Verification items for the finished model (mm, model axes). A direction names the side the tool comes from. Give positions to 0.01 mm unless a question says otherwise; leave off trailing zeros. Order: outer loops, then holes, each group sorted by start corner. A loop starts at its lowest first (then second) coordinate and runs counter-clockwise, first axis right, second up. Notation, with made-up numbers: M 3,62 L 24,62 A13 cw 24,72 Z; hole C 29,-13.5 d9. An arc over 180 degrees is marked long. Answer as a JSON object with one key per item and string values.
Autodesk Fusion 360 part; units mm, degrees
sketch "Boceto1" plane through (0, 0, 0) normal (1, 0, 0) x (0, 1, 0)
  line L0 (7.5, 35) -> (-7.5, 35)
  line L1 (-7.5, 35) -> (-7.5, -35)
  line L2 (-7.5, -35) -> (7.5, -35)
  line L3 (7.5, -35) -> (7.5, 35)
  line L4 (7.5, 35) -> (-7.5, -35) construction
  line L5 (-7.5, 35) -> (7.5, -35) construction
  circle A0 centre (0, 30) radius 2
  circle A1 centre (0, -30) radius 2
  line L6 (0, 35) -> (0, -35) construction
  dimension "d1" = 15
  dimension "d2" = 70
  dimension "d3" = 4
  dimension "d4" = 4
  dimension "d5" = 60
  dimension "d6" = 30
extrude "Extruir1" add sketch "Boceto1" along normal blind 3
sketch "Boceto2" plane through (3, 0, 0) normal (1, 0, 0) x (0, 1, 0)
  circle A0 centre (0, 30) radius 2
  circle A1 centre (0, -30) radius 2
  line L0 (7.5, -35) -> (7.5, 35)
  line L1 (7.5, 35) -> (-7.5, 35)
  line L2 (-7.5, 35) -> (-7.5, -35)
  line L3 (-7.5, -35) -> (7.5, -35)
  line L4 (3.25, 20) -> (-3.25, 20)
  line L5 (-3.25, 20) -> (-3.25, -20)
  line L6 (-3.25, -20) -> (3.25, -20)
  line L7 (3.25, -20) -> (3.25, 20)
  line L8 (3.25, 20) -> (-3.25, -20) construction
  line L9 (-3.25, 20) -> (3.25, -20) construction
  dimension "d9" = 6.5
  dimension "d10" = 40
extrude "Extruir2" add sketch "Boceto2" along normal blind 15 contours L4 L5 L6 L7
fillet "Empalme1" radius 2.5 4 edges at (3, 3.25, 0) (3, 0, -20) (3, -3.25, 0) (3, 0, 20)
Q1. Gauge pin test, flat ends, axial feed: pin 1 Ø4.5 at (y, z) = (0, 30) entering from +X; pin 2 Ø6 at (x, y) = (6.5, -2) entering from +Z; pin 3 Ø6 at (x, z) = (10.5, 6.5) entering from +Y. Record the tip position at first contact, or that the pin passes through.
Resolved:
{"pin 1": "stops at x = 3", "pin 2": "stops at z = 21", "pin 3": "stops at y = 3.25"}
Q2. Section check A-A on z = 30. Record the cut outline in (x, y), then the cut area to 3 significant figures.
Resolved:
{"outline": "M 0,-7.5 L 3,-7.5 L 3,-2 L 0,-2 Z; M 0,2 L 3,2 L 3,7.5 L 0,7.5 Z", "area": "33.0 mm²"}
Q3. Section check D-D on z = -5.5. Record the cut outline in (x, y).
Resolved:
{"outline": "M 0,-7.5 L 3,-7.5 L 3,-5.75 A2.5 cw 5.5,-3.25 L 18,-3.25 L 18,3.25 L 5.5,3.25 A2.5 cw 3,5.75 L 3,7.5 L 0,7.5 Z"}
Q4. Section check B-B on y = 0. Record the cut outline in (x, z).
Resolved:
{"outline": "M 0,-35 L 3,-35 L 3,-32 L 0,-32 Z; M 0,-28 L 3,-28 L 3,-22.5 A2.5 cw 5.5,-20 L 18,-20 L 18,20 L 5.5,20 A2.5 cw 3,22.5 L 3,28 L 0,28 Z; M 0,32 L 3,32 L 3,35 L 0,35 Z"}
Q5. Release check for a two-part mould opening along Z. For faces 1 (the face through (12, -3.25, 0)), 2 (the face through (1, 0, 32)), 3 (the face through (12, 0, 20)) record: +Z half, -Z half, draft (parallel to the pull), parting line (faces both ways), or undercut.
Resolved:
{"face 1": "draft", "face 2": "undercut", "face 3": "+Z half"}
Q6. Section check C-C on x = 1.25. Record the cut outline in (y, z), then the cut area to 3 significant figures.
Resolved:
{"outline": "M -7.5,-35 L 7.5,-35 L 7.5,35 L -7.5,35 Z; hole C 0,-30 d4; hole C 0,30 d4", "area": "1,020 mm²"}
Q7. Material ranges on L1, parallel to Z at x = 1.4, y = 0; L2, parallel to Z at x = 9.5, y = 2; L3, parallel to Y at x = 10.25, z = -15, recorded low to high.
Resolved:
{"L1": "z = -35 to -32, -28 to 28, 32 to 35", "L2": "z = -20 to 20", "L3": "y = -3.25 to 3.25"}
Q8. Tool access check on faces 4 (the face through (12, 3.25, 0)), 5 (the face through (1, 7.5, 0)), 6 (the face through (12, 0, -20)). Record the directions out of +Z, -Z, +X, -X, +Y, -Y that give a thin tool (end or side, any length) a straight path to the whole face; none if there is none.
Resolved:
{"face 4": "+Z, -Z, +X, +Y", "face 5": "+Z, -Z, +X, -X, +Y", "face 6": "-Z, +X, +Y, -Y"}
